```python
from build123d import *

# Parameters (mm, degrees)
F0_W     = 300
F0_H     = 110
F1_DEPTH = 25
F2_R     = 5
F3_DEPTH = 12
F4_R     = 5


with BuildPart() as f1:
    # F0 (on Top) → F1 (new body)
    with BuildSketch(Plane.XY):
        with Locations((-150, 55)):
            Rectangle(F0_W, F0_H)
    extrude(amount=F1_DEPTH)

    # F2 (on face) → F3 (cut)
    with BuildSketch(Plane.XY.offset(25)):
        with Locations((-262.5, 90)):
            Circle(F2_R)
        with Locations((-262.5, 20)):
            Circle(F2_R)
        with Locations((-37.5, 90)):
            Circle(F2_R)
        with Locations((-37.5, 20)):
            Circle(F2_R)
    extrude(amount=-F3_DEPTH, mode=Mode.SUBTRACT)

    # F4
    f4_edges = [f1.edges().sort_by_distance(p)[0] for p in [
        (0, 110, 12.5),
        (-300, 110, 12.5),
        (-150, 110, 0),
        (-150, 110, 25),
        (-300, 0, 12.5),
        (-300, 55, 0),
        (-300, 55, 25),
        (0, 0, 12.5),
        (-150, 0, 0),
        (-150, 0, 25),
        (0, 55, 0),
        (0, 55, 25),
    ]]
    fillet(f4_edges, radius=F4_R)


solid = f1.part
```
Could you check a few things on this model? Use its own coordinates, in mm. A direction names the side the tool comes from. Round coordinates to 2 decimals unless told otherwise and drop trailing zeros. Write each loop counter-clockwise with the first axis right and the second up, starting at its lowest first coordinate (ties: lowest second). Pieces come first, ordered by that corner, then holes. Notation, with made-up numbers: M 3.25,-33 L 44.25,-33 A24 cw 44.25,3 Z; hole C 84,27.5 d2. An arc over 180 degrees is marked long. Answer in a Markdown table with one row per item. Add a question column.
Q1. Imagine slicing it at A-A (x = -37.5). Please give me the cut outline in (y, z).
Q2. On a 3-axis mill with a long thin cutter (end or side, diameter ignored), from which of +Z, -Z, +X, -X, +Y, -Y can I reach the whole of each face in a straight line? I mean faces 4 (the cylindrical face through (-257.881, 18.085, 19.084)), 5 (the cylindrical face through (-299, 2, 13)). Say none if no direction works.
Q3. If we mould it in two halves opening along X, with no side actions, what happens to faces 1 (the cylindrical face through (-299, 56, 23)), 2 (the flat face through (-38, 90, 13)), 3 (the cylindrical face through (-148, 109, 2))? For each: +X half, -X half, draft (parallel to the pull), parting line (faces both ways), or undercut.
Q4. If I drill on line 1 (Y direction, x = -37.5, z = 17); line 2 (X direction, y = 25.5, z = 4.5); line 3 (Y direction, x = -37.5, z = 22.5), over which ranges is the centre line in solid material (lowest first)? Write a range as from..to.
Q5. Will this pin go through, and if not, where does the flat tip stop? pin 1 Ø5 at (x, y) = (-39.5, 19) entering from +Z.
Q6. Imagine slicing it at B-B (y = 90). Please give me the cut outline in (x, z), then the cut area to 3 significant figures.
Values:
| question | item | result |
|---|---|---|
| 1 | outline | M 0,5 A5 ccw 5,0 L 105,0 A5 ccw 110,5 L 110,20 A5 ccw 105,25 L 95,25 L 95,13 L 85,13 L 85,25 L 25,25 L 25,13 L 15,13 L 15,25 L 5,25 A5 ccw 0,20 Z |
| 2 | face 4 | +Z |
| 2 | face 5 | +Z, -Z, -X, -Y |
| 3 | face 1 | -X half |
| 3 | face 2 | undercut |
| 3 | face 3 | draft |
| 4 | line 1 | 0..15, 25..85, 95..110 |
| 4 | line 2 | -299.97..-0.03 |
| 4 | line 3 | 0.67..15, 25..85, 95..109.33 |
| 5 | pin 1 | z = 13 |
| 6 | outline | M -300,5 A5 ccw -295,0 L -5,0 A5 ccw 0,5 L 0,20 A5 ccw -5,25 L -32.5,25 L -32.5,13 L -42.5,13 L -42.5,25 L -257.5,25 L -257.5,13 L -267.5,13 L -267.5,25 L -295,25 A5 ccw -300,20 Z |
| 6 | area | 7,240 mm^2 |
